```python
from build123d import *

# Parameters (mm, degrees)
CUT_EXTRUDE3_DEPTH           = 60
CUT_EXTRUDE5_DEPTH           = 2
CUT_EXTRUDE5_DEPTH_BACK      = 30
SKETCH9_R                    = 38
SKETCH9_R_2                  = 23
SKETCH19_W                   = 12
SKETCH19_H                   = 36.5
CUT_REVOLVE2_ANGLE           = 65
CUT_REVOLVE2_OTHER_WAY_ANGLE = 65
SKETCH21_W                   = 3.25
SKETCH21_H                   = 4
BOSS_EXTRUDE3_DEPTH          = 1.35
CIRPATTERN1_COUNT            = 5
CUT_EXTRUDE9_START           = -5
CUT_EXTRUDE9_DEPTH           = 5
SKETCH23_R                   = 10.5
CUT_EXTRUDE10_DEPTH          = 10
SKETCH24_W                   = 15
SKETCH24_H                   = 8
BOSS_EXTRUDE4_DEPTH          = 8
SKETCH26_W                   = 10
SKETCH26_H                   = 6
CUT_EXTRUDE11_DEPTH          = 10
SKETCH27_W                   = 4
SKETCH27_H                   = 5
CUT_EXTRUDE12_DEPTH          = 5
CUT_EXTRUDE14_DEPTH          = 2
CUT_EXTRUDE14_DEPTH_BACK     = 30
SKETCH29_R                   = 1
CUT_EXTRUDE15_DEPTH          = 15
FILLET1_R                    = 6
FILLET2_R                    = 8
INTERSECT2_START             = 13
INTERSECT2_DEPTH             = 50.427876097


# Read off the part's stored shape, not the designer's step: Cut-Extrude9, Intersect2
with BuildPart() as part:
    # Sketch1 → Revolve1 (revolve)
    with BuildSketch(Plane.XY, mode=Mode.PRIVATE) as revolve1_sk:
        with BuildLine():
            Line((0, 63.427876097), (32, 63.427876097))
            ThreePointArc((32, 63.427876097), (37.656854249, 61.084730346), (40, 55.427876097))
            Line((40, 55.427876097), (40, 28.846818009))
            ThreePointArc((40, 28.846818009), (38.792081772, 24.082439968), (35.460140376, 20.469057744))
            Line((35.460140376, 20.469057744), (28.539859624, 15.958818353))
            ThreePointArc((28.539859624, 15.958818353), (25.207918228, 12.345436129), (24, 7.581058088))
            Line((24, 7.581058088), (24, 3.25))
            Line((24, 3.25), (24.35, 3))
            Line((24.35, 3), (24.35, 0))
            Line((24.35, 0), (22.5, 0))
            Line((22.5, 0), (22.5, 12.5))
            ThreePointArc((22.5, 12.5), (22.353553391, 12.853553391), (22, 13))
            Line((22, 13), (0, 13))
            Line((0, 13), (0, 63.427876097))
        make_face()
    revolve(revolve1_sk.sketch.rotate(Axis((0, 0, 0), (0, 1, 0)), 90), axis=Axis((0, 0, 0), (0, 1, 0)))

    # Sketch11 → Cut-Extrude3 (cut)
    with BuildSketch(Plane(origin=(0, 13, 0), x_dir=(-1, 0, 0), z_dir=(0, -1, 0))):
        with BuildLine():
            Line((-21, 0), (21, 0))
            ThreePointArc((21, 0), (0, 21), (-21, 0))
        make_face()
    extrude(amount=-CUT_EXTRUDE3_DEPTH, mode=Mode.SUBTRACT)

    # Sketch9 → Cut-Extrude5 (cut, two sides: drawn at the far end of the back side and taken through both)
    with BuildSketch(Plane(origin=(0, 55.427876097, 0), x_dir=(1, 0, 0), z_dir=(0, 1, 0)).offset(-CUT_EXTRUDE5_DEPTH_BACK)):
        with Locations(Location((0, 0, 0), (0, 0, 270))):
            Circle(SKETCH9_R)
        with Locations(Location((0, 0, 0), (0, 0, 270))):
            Circle(SKETCH9_R_2, mode=Mode.SUBTRACT)
    extrude(amount=CUT_EXTRUDE5_DEPTH + CUT_EXTRUDE5_DEPTH_BACK, mode=Mode.SUBTRACT)

    # Sketch19 → Cut-Revolve2 (revolve, cut)
    with BuildSketch(Plane(origin=(0, 0, 0), x_dir=(0, 0, -1), z_dir=(1, 0, 0))):
        with Locations((-41.064715832, 37.177876097)):
            Rectangle(SKETCH19_W, SKETCH19_H)
    revolve(axis=Axis((0, 0, 0), (0, 1, 0)), revolution_arc=CUT_REVOLVE2_ANGLE, mode=Mode.SUBTRACT)

    # Sketch19 → Cut-Revolve2 other way (revolve, cut)
    with BuildSketch(Plane(origin=(0, 0, 0), x_dir=(0, 0, -1), z_dir=(1, 0, 0))):
        with Locations((-41.064715832, 37.177876097)):
            Rectangle(SKETCH19_W, SKETCH19_H)
    revolve(axis=Axis((0, 0, 0), (0, -1, 0)), revolution_arc=CUT_REVOLVE2_OTHER_WAY_ANGLE, mode=Mode.SUBTRACT)

    # Sketch21 → Boss-Extrude3 (add)
    with BuildSketch(Plane(origin=(0, 0, 22.5), x_dir=(-1, 0, 0), z_dir=(0, 0, -1))):
        with Locations((0, 2)):
            Rectangle(SKETCH21_W, SKETCH21_H)
    boss_extrude3 = extrude(amount=BOSS_EXTRUDE3_DEPTH)

    # CirPattern1: Boss-Extrude3 ×5 about axis
    cirpattern1_axis = Axis((0, 0, 0), (0, 1, 0))
    for i in range(1, CIRPATTERN1_COUNT):
        add(boss_extrude3.rotate(cirpattern1_axis, i * 360 / CIRPATTERN1_COUNT))

    # Cut-Extrude9 outline → Cut-Extrude9 (cut)
    with BuildSketch(Plane(origin=(0, 63.427876097, 0), x_dir=(1, 0, 0), z_dir=(0, 1, 0)).offset(CUT_EXTRUDE9_START)):
        with BuildLine():
            ThreePointArc((40, 0), (0, 40), (-40, 0))
            Line((-40, 0), (-21, 0))
            ThreePointArc((-21, 0), (0, 21), (21, 0))
            Line((21, 0), (40, 0))
        make_face()
    extrude(amount=CUT_EXTRUDE9_DEPTH, mode=Mode.SUBTRACT)

    # Sketch23 → Cut-Extrude10 (cut)
    with BuildSketch(Plane(origin=(0, 0, -40), x_dir=(-1, 0, 0), z_dir=(0, 0, -1))):
        with Locations((0, 42.137876097)):
            Circle(SKETCH23_R)
    extrude(amount=-CUT_EXTRUDE10_DEPTH, mode=Mode.SUBTRACT)

    # Sketch24 → Boss-Extrude4 (add)
    with BuildSketch(Plane(origin=(0, 58.427876097, 0), x_dir=(1, 0, 0), z_dir=(0, 1, 0))):
        with Locations((0, 30)):
            Rectangle(SKETCH24_W, SKETCH24_H)
    extrude(amount=-BOSS_EXTRUDE4_DEPTH)

    # Sketch26 → Cut-Extrude11 (cut)
    with BuildSketch(Plane(origin=(0, 58.427876097, 0), x_dir=(1, 0, 0), z_dir=(0, 1, 0))):
        with Locations((0, 30)):
            Rectangle(SKETCH26_W, SKETCH26_H)
    extrude(amount=-CUT_EXTRUDE11_DEPTH, mode=Mode.SUBTRACT)

    # Sketch27 → Cut-Extrude12 (cut)
    with BuildSketch(Plane(origin=(7.5, 0, 0), x_dir=(0, 0, -1), z_dir=(1, 0, 0))):
        with Locations((30, 53.927876097)):
            Rectangle(SKETCH27_W, SKETCH27_H)
    extrude(amount=-CUT_EXTRUDE12_DEPTH, mode=Mode.SUBTRACT)

    # Sketch28 → Cut-Extrude14 (cut, two sides: drawn at the far end of the back side and taken through both)
    with BuildSketch(Plane(origin=(0, 55.427876097, 0), x_dir=(1, 0, 0), z_dir=(0, 1, 0)).offset(-CUT_EXTRUDE14_DEPTH_BACK)):
        with BuildLine():
            Line((-22.912878475, -2), (22.912878475, -2))
            ThreePointArc((22.912878475, -2), (0, -23), (-22.912878475, -2))
        make_face()
    extrude(amount=CUT_EXTRUDE14_DEPTH + CUT_EXTRUDE14_DEPTH_BACK, mode=Mode.SUBTRACT)

    # Sketch29 → Cut-Extrude15 (cut)
    with BuildSketch(Plane(origin=(0, 0, 0), x_dir=(-1, 0, 0), z_dir=(0, 0, -1))):
        with Locations((-30.416198487, 60.927876097)):
            Circle(SKETCH29_R)
        with Locations((30.416198487, 60.927876097)):
            Circle(SKETCH29_R)
        with Locations((0, 60.927876097)):
            Circle(SKETCH29_R)
    extrude(amount=-CUT_EXTRUDE15_DEPTH, mode=Mode.SUBTRACT)

    # Fillet1
    fillet1_edges = [part.edges().sort_by_distance(p)[0] for p in [
        (21, 35.713938048, 0),
        (-21, 35.713938048, 0),
    ]]
    fillet(fillet1_edges, radius=FILLET1_R)

    # Fillet2
    fillet2_edges = [part.edges().sort_by_distance(p)[0] for p in [
        (-22.912878475, 41.427876097, 2),
        (22.912878475, 41.427876097, 2),
    ]]
    fillet(fillet2_edges, radius=FILLET2_R)

    # Intersect2 outline → Intersect2 (cut)
    with BuildSketch(Plane(origin=(0, 0, 0), x_dir=(1, 0, 0), z_dir=(0, 1, 0)).offset(INTERSECT2_START)):
        with BuildLine():
            Line((-37.080992435, -15), (-42, -15))
            Line((-42, -15), (-42, -42))
            Line((-42, -42), (42, -42))
            Line((42, -42), (42, -15))
            Line((42, -15), (37.080992435, -15))
            ThreePointArc((37.080992435, -15), (0, 40), (-37.080992435, -15))
        make_face()
        with BuildLine():
            ThreePointArc((-13.747727085, 0), (-18.767687244, 2.713664655), (-19.246817919, 8.4))
            ThreePointArc((-19.246817919, 8.4), (0, 21), (19.246817919, 8.4))
            ThreePointArc((19.246817919, 8.4), (18.767687244, 2.713664655), (13.747727085, 0))
            Line((13.747727085, 0), (-13.747727085, 0))
        make_face(mode=Mode.SUBTRACT)
    extrude(amount=INTERSECT2_DEPTH, mode=Mode.SUBTRACT)


solid = part.part
```
For this review, take the finished solid that the model builds, in its own axes (mm). A direction names the side the tool comes from. Round coordinates to 2 decimals unless told otherwise and drop trailing zeros. Order: outer loops, then holes, each group sorted by start corner. A loop starts at its lowest first (then second) coordinate and runs counter-clockwise, first axis right, second up.
Q1. We need section C-C, the plane y = 5. Give the boundary of the cut face in (x, z).
Findings below:
outline: circle Ø48 at (0, 0); hole circle Ø45 at (0, 0)
Q2. Insertion check: P1, Ø1.5, axis at x = -12.5, z = -17, coming from the +Y side; P2, Ø5, axis at y = 4.5, z = 15.5, coming from the -X side; P3, Ø3, axis at x = -19.5, y = 11, coming from the +Z side. Each pin has a flat end and moves straight along its axis. Give the tip position at first contact, or say it passes through.
Findings below:
P1: stops at y = 4
P2: stops at x = -20.27
P3: stops at z = 17.01
Q3. Wall thickness on line 1 (X direction, y = 6, z = 0); line 2 (Z direction, x = -16, y = 7.75); line 3 (Z direction, x = 19.5, y = 1.25): over which ranges is each line inside the solid? List them lowest first.
Findings below:
line 1: x = -24 to -22.5, 22.5 to 24
line 2: z = -17.89 to -15.82, 15.82 to 17.89
line 3: z = -14.58 to -11.22, 11.22 to 14.58
Q4. Machinability: for faces 1 (the flat face through (-21.24, 1.972, 5.193)), 2 (the flat face through (13, 4, -18)), 3 (the flat face through (-20.108, 2.028, 6.557)), which of the approach directions +Z, -Z, +X, -X, +Y, -Y give a long, thin tool a straight path to every point of the face, cutting with its end or side? Answer none if there is none.
Findings below:
face 1: -Y
face 2: none
face 3: +Y, -Y
Q5. We need section B-B, the plane x = 0. Give the boundary of the cut face in (y, z), plus the area to 3 significant figures.
Findings below:
outline: (0, -24.35) - (3, -24.35) - (3.25, -24) - (7.58, -24) arc R10 cw to (13, -25.6) - (13, -22) arc R0.5 cw to (12.5, -22.5) - (0, -22.5) - close; (0, 21.15) - (4, 21.15) - (4, 22.5) - (12.5, 22.5) arc R0.5 cw to (13, 22) - (13, 25.6) arc R10 cw to (7.58, 24) - (3.25, 24) - (3, 24.35) - (0, 24.35) - close
area: 52.3 mm2
Q6. We need section A-A, the plane z = 0. Give the boundary of the cut face in (x, y), plus the area to 3 significant figures.
Findings below:
outline: (-25.6, 13) arc R10 cw to (-24, 7.58) - (-24, 3.25) - (-24.35, 3) - (-24.35, 0) - (-22.5, 0) - (-22.5, 12.5) arc R0.5 cw to (-22, 13) - close; (22, 13) arc R0.5 cw to (22.5, 12.5) - (22.5, 0) - (24.35, 0) - (24.35, 3) - (24, 3.25) - (24, 7.58) arc R10 cw to (25.6, 13) - close
area: 46.9 mm2
Q7. Mouldability with a two-part tool opening along Z and no side actions: class faces 4 (the cylindrical face through (14.82, 1.48, 19.32)), 5 (the flat face through (-1.625, 2, 22)), 6 (the flat face through (-8, 13, -21)), 7 (the flat face through (20.122, 2.028, 6.514)) as pulls with the +Z half, pulls with the -Z half, needs draft (parallel to the pull), parting line crosses it, or undercut.
Findings below:
face 4: parting line crosses it
face 5: undercut
face 6: needs draft
face 7: undercut
Q8. We need section D-D, the plane y = 11.75. Give the boundary of the cut face in (x, z), plus the area to 3 significant figures.
Findings below:
outline: circle Ø49.82 at (0, 0); hole circle Ø45 at (0, 0)
area: 359 mm2
